Read the model definition and answer for the solid it produces. Units are mm, in the model's axes. A direction names the side the tool comes from. Round coordinates to 2 decimals unless told otherwise and drop trailing zeros. Order: outer loops, then holes, each group sorted by start corner. A loop starts at its lowest first (then second) coordinate and runs counter-clockwise, first axis right, second up. Notation, with made-up numbers: (4.25, 15) -> (14.25, 15) arc R33 ccw to (14.25, 43) -> close; hole circle Ø10 at (43, 41.25). An arc over 180 degrees is marked (long way). Use a Markdown table: item, result. Add a question column.
1. Given pin 1 (5 mm diameter, centred on x = -4.5, z = -83, fed in from -Y); pin 2 (8 mm diameter, centred on x = 47, y = -16, fed in from -Z), each flat-ended and moving along its own axis, determine where each tip first touches the part or whether it passes through.
2. For faces 1 (the face through (-105.04, 9.86, -103.95)), 2 (the face through (2, 0, -26)), determine the directions among +Z, -Z, +X, -X, +Y, -Y from which every point of the face is accessible in a straight line to the end or side of a thin tool.
3. Consider L1, parallel to Y at x = 82, z = 29; L2, parallel to Z at x = 15.5, y = -44; L3, parallel to Z at x = 72, y = 3. Determine where each line is inside the solid, lowest interval first. Write a range as [from, to].
4. Section A-A, the plane x = 47 is taken. Give the vertices of the cut face in (y, z), then the cut area to 3 significant figures.
5. Section C-C, the plane y = -13 is taken. Give the vertices of the cut face in (x, z).
6. Section B-B, the plane z = 27 is taken. Give the vertices of the cut face in (x, y).
7. Section D-D, the plane x = 97 is taken. Give the vertices of the cut face in (y, z), then the cut area to 3 significant figures.
```python
from build123d import *

# Parameters (mm, degrees)
BOSS_EXTRUDE1_DEPTH = 20
SKETCH2_W           = 250
SKETCH2_H           = 50
BOSS_EXTRUDE2_DEPTH = 50
FILLET1_R           = 10


with BuildPart() as part:
    # Sketch1 → Boss-Extrude1 (new body)
    with BuildSketch(Plane(origin=(0, 0, 0), x_dir=(1, 0, 0), z_dir=(0, 1, 0))):
        with BuildLine():
            Line((-55, 125), (55, 125))
            ThreePointArc((55, 125), (104.497474683, 104.497474683), (125, 55))
            Line((125, 55), (125, -125))
            Line((125, -125), (-125, -125))
            Line((-125, -125), (-125, 55))
            ThreePointArc((-125, 55), (-104.497474683, 104.497474683), (-55, 125))
        make_face()
    extrude(amount=BOSS_EXTRUDE1_DEPTH)

    # Sketch2 → Boss-Extrude2 (add)
    with BuildSketch(Plane.XZ):
        with Locations((0, 100)):
            Rectangle(SKETCH2_W, SKETCH2_H)
    extrude(amount=BOSS_EXTRUDE2_DEPTH)

    # Fillet1
    fillet1_edges = [part.edges().sort_by_distance(p)[0] for p in [
        (0, 20, 125),
    ]]
    fillet(fillet1_edges, radius=FILLET1_R)


solid = part.part
```
Verdict:
| question | item | result |
|---|---|---|
| 1 | pin 1 | stops at y = 0 |
| 1 | pin 2 | stops at z = 75 |
| 2 | face 1 | -Z, -X, +Y, -Y |
| 2 | face 2 | -Z, +X, -X, -Y |
| 3 | L1 | y = [0, 20] |
| 3 | L2 | z = [75, 125] |
| 3 | L3 | z = [-122.9, 125] |
| 4 | outline | (-50, 75) -> (0, 75) -> (0, -125) -> (20, -125) -> (20, 115) arc R10 ccw to (10, 125) -> (-50, 125) -> close |
| 4 | area | 7,480 mm2 |
| 5 | outline | (-125, 75) -> (125, 75) -> (125, 125) -> (-125, 125) -> close |
| 6 | outline | (-125, 0) -> (125, 0) -> (125, 20) -> (-125, 20) -> close |
| 7 | outline | (-50, 75) -> (0, 75) -> (0, -111) -> (20, -111) -> (20, 115) arc R10 ccw to (10, 125) -> (-50, 125) -> close |
| 7 | area | 7,200 mm2 |
